Could you check a few things on this model? Use its own coordinates, in mm. A direction names the side the tool comes from. Coordinates: 2 decimals unless noted, no trailing zeros. Loops run counter-clockwise (first coordinate to the right, second up) from the corner with the lowest first, then second, coordinate; pieces in that order, holes last. Notation, with made-up numbers: M 24,34 L 62,34 A19 cw 62,63 Z; hole C 54,10 d11. An arc over 180 degrees is marked long. Return JSON: item names as keys, results as strings. Group by question number.
from build123d import *

# Parameters (mm, degrees)
F2_DEPTH = 76.2
F3_W     = 30.48
F3_H     = 30.48
F4_DEPTH = 5.08


with BuildPart() as f2:
    # F0 (on Top) → F2 (new body)
    with BuildSketch(Plane.XY):
        Polygon((-30.320511, 87.794254), (-68.420511, 21.803118), (-30.320511, -44.188018), (45.879489, -44.188018), (83.979489, 21.803118), (45.879489, 87.794254), align=None)
        Polygon((-27.387572, -39.108018), (-62.554632, 21.803118), (-27.387572, 82.714254), (42.94655, 82.714254), (78.11361, 21.803118), (42.94655, -39.108018), (-7.85345, -39.108018), align=None, mode=Mode.SUBTRACT)
    extrude(amount=F2_DEPTH)

    # F3 (on face) → F4 (cut)
    with BuildSketch(Plane.XZ.offset(44.188018)):
        with Locations((7.779489, 40.64)):
            Rectangle(F3_W, F3_H)
    extrude(amount=-F4_DEPTH, mode=Mode.SUBTRACT)


solid = f2.part
(1) Will these pins go through, and if not, where does the flat tip stop? P1, Ø1.5, axis at y = 29.5, z = 66.5, coming from the +X side; P2, Ø1, axis at y = 14.5, z = 37, coming from the +X side; P3, Ø1.5, axis at y = 55.5, z = 31, coming from the +X side.
(2) If I drill on L1, parallel to Y at x = -26, z = 33; L2, parallel to X at y = 60, z = 47; L3, parallel to Y at x = 53, z = 43, over which ranges is the centre line in solid material (lowest first)? Write a range as [from, to].
(3) Imagine slicing it at C-C, the plane y = -19. Write out the boundary of the cut face in (x, z), then the cut area to 3 significant figures.
(4) Imagine slicing it at D-D, the plane z = 45. Write out the boundary of the cut face in (x, y), then the cut area to 3 significant figures.
(5) We'd pull the mould along Z, two halves only. Please class faces 1 (the face through (64, 47, 76.2)), 2 (the face through (64, 47, 0)), 3 (the face through (60.776, -8.226, 37.567)), 4 (the face through (23.019, -42, 40)): +Z half, -Z half, draft (parallel to the pull), parting line (faces both ways), or undercut.
(6) Imagine slicing it at A-A, the plane x = 28.5. Write out the boundary of the cut face in (y, z), then the cut area to 3 significant figures.
(7) For faces 5 (the face through (60.28, 52.69, 37.57)), 6 (the face through (-7.461, -42, 40)), 7 (the face through (65.196, 54.337, 37.567)), which set-ups out of +Z, -Z, +X, -X, +Y, -Y let a thin tool reach every point of the face, with its end or its side?
(8) Imagine slicing it at B-B, the plane z = 67. Write out the boundary of the cut face in (x, y), then the cut area to 3 significant figures.
Checks:
{
 "1": {"P1": "x = 79.97", "P2": "x = 80.05", "P3": "x = 64.96"},
 "2": {"L1": "[-44.19, -39.11], [82.71, 87.79]", "L2": "[-46.37, -40.5], [56.06, 61.93]", "L3": "[-31.85, -21.69], [65.3, 75.46]"},
 "3": {"outline": "M -44.86,0 L -39,0 L -39,76.2 L -44.86,76.2 Z; M 54.56,0 L 60.42,0 L 60.42,76.2 L 54.56,76.2 Z", "area": "894 mm²"},
 "4": {"outline": "M -68.42,21.8 L -30.32,-44.19 L -7.46,-44.19 L -7.46,-39.11 L -27.39,-39.11 L -62.55,21.8 L -27.39,82.71 L 42.95,82.71 L 78.11,21.8 L 42.95,-39.11 L 23.02,-39.11 L 23.02,-44.19 L 45.88,-44.19 L 83.98,21.8 L 45.88,87.79 L -30.32,87.79 Z", "area": "2,080 mm²"},
 "5": {"face 1": "+Z half", "face 2": "-Z half", "face 3": "draft", "face 4": "undercut"},
 "6": {"outline": "M -44.19,0 L -39.11,0 L -39.11,76.2 L -44.19,76.2 Z; M 82.71,0 L 87.79,0 L 87.79,76.2 L 82.71,76.2 Z", "area": "774 mm²"},
 "7": {"face 5": "+Z, -Z", "face 6": "-Y", "face 7": "+Z, -Z, +X, +Y"},
 "8": {"outline": "M -68.42,21.8 L -30.32,-44.19 L 45.88,-44.19 L 83.98,21.8 L 45.88,87.79 L -30.32,87.79 Z; hole M -62.55,21.8 L -27.39,-39.11 L 42.95,-39.11 L 78.11,21.8 L 42.95,82.71 L -27.39,82.71 Z", "area": "2,230 mm²"}
}
